```python
from build123d import *

# Parameters (mm, degrees)
SKETCH007_W     = 30.1
SKETCH007_H     = 30.1
SKETCH007_W_2   = 20.1
SKETCH007_H_2   = 20.1
PAD005_DEPTH    = 10
SKETCH008_W     = 30.1
SKETCH008_H     = 30.1
SKETCH008_R     = 2.75
PAD006_DEPTH    = 3
PAD007_DEPTH    = 2
CHAMFER003_SIZE = 4


with BuildPart() as part:
    # Sketch007 → Pad005 (new body)
    with BuildSketch(Plane.XY):
        Rectangle(SKETCH007_W, SKETCH007_H)
        Rectangle(SKETCH007_W_2, SKETCH007_H_2, mode=Mode.SUBTRACT)
    extrude(amount=-PAD005_DEPTH)

    # Sketch008 → Pad006 (join)
    with BuildSketch(Plane.XY):
        Rectangle(SKETCH008_W, SKETCH008_H)
        Circle(SKETCH008_R, mode=Mode.SUBTRACT)
    extrude(amount=PAD006_DEPTH)

    # Sketch009 → Pad007 (join, symmetric)
    with BuildSketch(Plane.XZ):
        Polygon((16.05, 3), (15.55, 1), (17.05, -3), (15.05, -3), (15.05, -10), (20.05, -5), (20.05, 3), align=None)
    extrude(amount=PAD007_DEPTH, both=True)

    # Chamfer003
    chamfer003_edges = [part.edges().sort_by_distance(p)[0] for p in [
        (15.05, -15.05, 1.5),
        (15.05, -15.05, -5),
        (-15.05, -15.05, 1.5),
        (-15.05, -15.05, -5),
        (15.05, 15.05, 1.5),
        (15.05, 15.05, -5),
        (-15.05, 15.05, 1.5),
        (-15.05, 15.05, -5),
    ]]
    chamfer(chamfer003_edges, length=CHAMFER003_SIZE)


with BuildPart() as part_1:
    # Body003 placement: moved
    add(part.part.moved(Location((0, 0, 100))))


solid = part_1.part
```
CAD build for the part. Positions are in the model's coordinates, mm. A direction names the side the tool comes from. Round coordinates to 2 decimals unless told otherwise and drop trailing zeros. Write each loop counter-clockwise with the first axis right and the second up, starting at its lowest first coordinate (ties: lowest second). Pieces come first, ordered by that corner, then holes.
Item 1: Tool access for faces 1 (the flat face through (-2.4, 2.4, 100)), 2 (the flat face through (18, 2, 97)), 3 (the flat face through (18, -2, 97)), 4 (the flat face through (-15.05, 0, 96)), 5 (the flat face through (16.3, 0, 99)): list every direction of +Z, -Z, +X, -X, +Y, -Y with a clear straight run to the whole face (end or side of a thin tool).
Filled in:
face 1: -Z
face 2: +Z, -Z, +X, +Y
face 3: +Z, -Z, +X, -Y
face 4: +Z, -Z, -X, +Y, -Y
face 5: +Y, -Y
Item 2: Band-saw the part on A-A on x = 0. Write the cut outline in (y, z).
Filled in:
outline: (-15.05, 90) - (-10.05, 90) - (-10.05, 100) - (-2.75, 100) - (-2.75, 103) - (-15.05, 103) - close; (2.75, 100) - (10.05, 100) - (10.05, 90) - (15.05, 90) - (15.05, 103) - (2.75, 103) - close
Item 3: Band-saw the part on C-C on y = 9.5. Write the cut outline in (x, z), then the cut area to 3 significant figures.
Filled in:
outline: (-15.05, 90) - (-10.05, 90) - (-10.05, 100) - (10.05, 100) - (10.05, 90) - (15.05, 90) - (15.05, 103) - (-15.05, 103) - close
area: 190 mm2
Item 4: Band-saw the part on B-B on y = 0. Write the cut outline in (x, z).
Filled in:
outline: (-15.05, 90) - (-10.05, 90) - (-10.05, 100) - (-2.75, 100) - (-2.75, 103) - (-15.05, 103) - close; (2.75, 100) - (10.05, 100) - (10.05, 90) - (15.05, 90) - (20.05, 95) - (20.05, 103) - (16.05, 103) - (15.55, 101) - (17.05, 97) - (15.05, 97) - (15.05, 103) - (2.75, 103) - close
Item 5: Drop flat-ended pins along their axis: pin 1 Ø1.6 at (x, y) = (16, 0) entering from +Z; pin 2 Ø2.5 at (x, z) = (18.5, 94.5) entering from -Y; pin 3 Ø6.5 at (x, y) = (0, 0) entering from -Z; pin 4 Ø5.5 at (x, z) = (17, 95) entering from +Y. Give the stop position or say it passes through.
Filled in:
pin 1: stops at z = 103
pin 2: stops at y = -2
pin 3: stops at z = 100
pin 4: stops at y = 11.85
Item 6: Drill centre lines: L1, parallel to Y at x = 7.5, z = 97; L2, parallel to Y at x = 0, z = 101.05. Where is each one in solid material? Low to high.
Filled in:
L1: y = -15.05 to -10.05, 10.05 to 15.05
L2: y = -15.05 to -2.75, 2.75 to 15.05
Item 7: Mould opens along Y. For faces 6 (the flat face through (-13, -13.1, 96.4)), 7 (the flat face through (0, 15.05, 96)), 8 (the flat face through (15.8, 0, 102)), 9 (the cylindrical face through (-0.596, -2.685, 101.479)) say: released by +Y, released by -Y, zero draft, split by the parting line, or undercut.
Filled in:
face 6: released by -Y
face 7: released by +Y
face 8: zero draft
face 9: undercut
